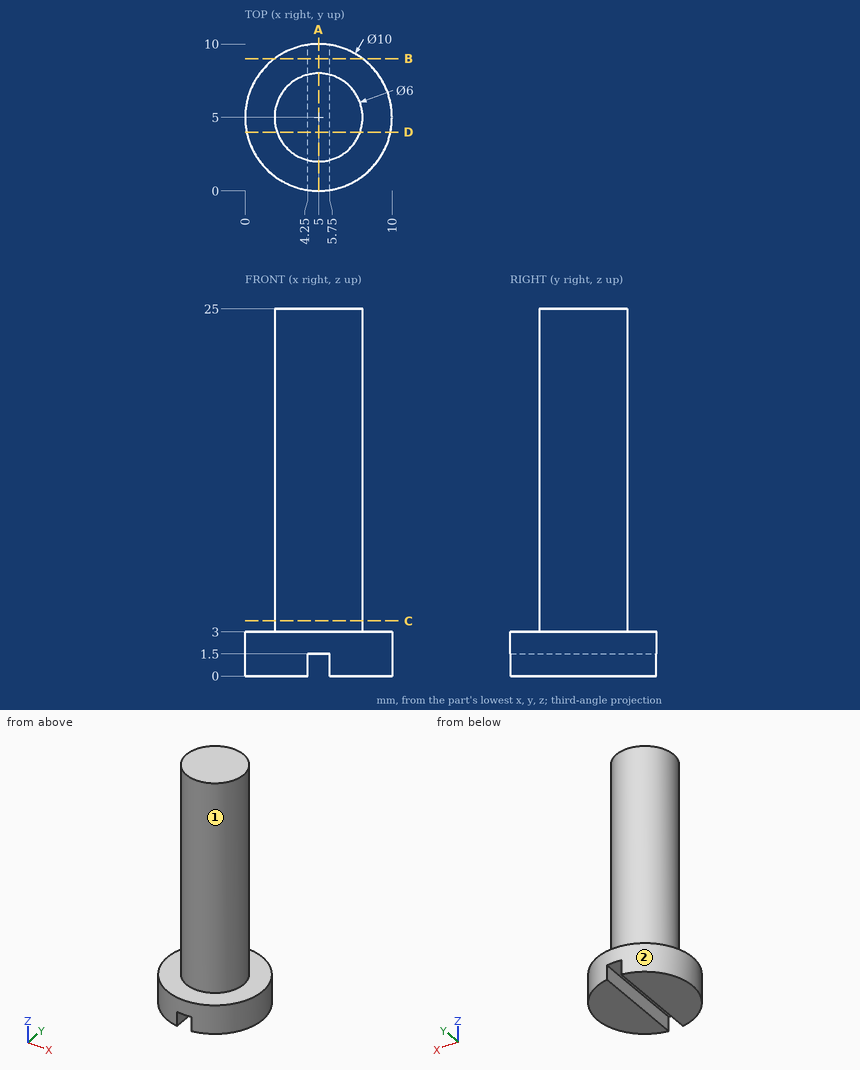
Can you work these out from the drawing? Everything is in mm from the part's minimum corner. A direction names the side the tool comes from. Coordinates: 2 decimals unless noted, no trailing zeros. Loops run counter-clockwise (first coordinate to the right, second up) from the corner with the lowest first, then second, coordinate; pieces in that order, holes last. Notation, with made-up numbers: M -19,89.5 L -5,89.5 A20 cw -5,96.5 Z; hole C -25,-8 d8. An arc over 180 degrees is marked long. Put each result on its own line as item: value. Start each with the question number.
(1) Suppose I cut it at B-B on y = 9. Please give me the cut outline in (x, z), then the cut area to 4 significant figures.
(2) I need wall thicknesses on line 1 (Z direction, x = 5.25, y = 3); line 2 (Z direction, x = 5.5, y = 0.5); line 3 (X direction, y = 6.5, z = 4.25). Which ranges of each line are inside material? Lowest first, please. Write a range as from..to.
(3) For the marked faces 1 and 2, which set-ups out of +Z, -Z, +X, -X, +Y, -Y let a thin tool reach every point of the face, with its end or its side?
(4) Suppose I cut it at A-A on x = 5. Please give me the cut outline in (y, z).
(5) Suppose I cut it at C-C on z = 3.75. Please give me the cut outline in (x, y).
(6) Suppose I cut it at D-D on y = 4. Please give me the cut outline in (x, z).
(7) Will these pins go through, and if not, where does the flat tip stop? P1, Ø3, axis at x = 1, z = 22, coming from the -Y side; P2, Ø3, axis at y = 5.5, z = 10.5, coming from the -X side; P3, Ø1.2, axis at x = 5.5, y = 3, coming from the -Z side; P4, Ø1.5, axis at y = 8, z = 16.5, coming from the -X side.
Solutions:
1. outline: M 2,0 L 4.25,0 L 4.25,1.5 L 5.75,1.5 L 5.75,0 L 8,0 L 8,3 L 2,3 Z
1. area: 15.75 mm2
2. line 1: z = 1.5..25
2. line 2: z = 1.5..3
2. line 3: x = 2.4..7.6
3. face 1: +Z
3. face 2: +Z, -Z
4. outline: M 0,1.5 L 10,1.5 L 10,3 L 8,3 L 8,25 L 2,25 L 2,3 L 0,3 Z
5. outline: C 5,5 d6
6. outline: M 0.1,0 L 4.25,0 L 4.25,1.5 L 5.75,1.5 L 5.75,0 L 9.9,0 L 9.9,3 L 7.83,3 L 7.83,25 L 2.17,25 L 2.17,3 L 0.1,3 Z
7. P1: stops at y = 3.34
7. P2: stops at x = 2
7. P3: stops at z = 0
7. P4: stops at x = 3.02
